```python
from build123d import *

# Parameters (mm, degrees)
EXTRUDE_1_DEPTH     = 4
SKETCH_3_R          = 5.9
EXTRUDE_2_DEPTH     = 1
SKETCH_4_R          = 2.15
CUT_EXTRUDE_1_DEPTH = 10.727281223
CHAMFER_1_SIZE      = 0.5


with BuildPart() as part:
    # Sketch 1 → Extrude 1 (new body)
    with BuildSketch(Plane.XY):
        Polygon((0, 4.618802154), (-4, 2.309401077), (-4, -2.309401077), (0, -4.618802154), (4, -2.309401077), (4, 2.309401077), align=None)
    extrude(amount=-EXTRUDE_1_DEPTH)

    # Sketch 2 → Cut-Revolve 1 (revolve, cut)
    with BuildSketch(Plane(origin=(0, 0, 0), x_dir=(0, 0, -1), z_dir=(1, 0, 0))):
        Polygon((0, 4.618802154), (0.35726559, 4.618802154), (0, 4), align=None)
        Polygon((4, 4), (3.64273441, 4.618802154), (4, 4.618802154), align=None)
    revolve(axis=Axis((0, 0, 0), (0, 0, -1)), mode=Mode.SUBTRACT)

    # Sketch 3 → Extrude 2 (add)
    with BuildSketch(Plane.XY):
        Circle(SKETCH_3_R)
    extrude(amount=EXTRUDE_2_DEPTH)

    # Sketch 4 → Cut-Extrude 1 (cut, through all)
    with BuildSketch(Plane(origin=(0, 0, -4), x_dir=(-1, 0, 0), z_dir=(0, 0, -1))):
        Circle(SKETCH_4_R)
    extrude(amount=-CUT_EXTRUDE_1_DEPTH, mode=Mode.SUBTRACT)

    # Chamfer 1
    chamfer_1_edges = [part.edges().sort_by_distance(p)[0] for p in [
        (2.15, 0, 1),
        (2.15, 0, -4),
    ]]
    chamfer(chamfer_1_edges, length=CHAMFER_1_SIZE)


solid = part.part
```
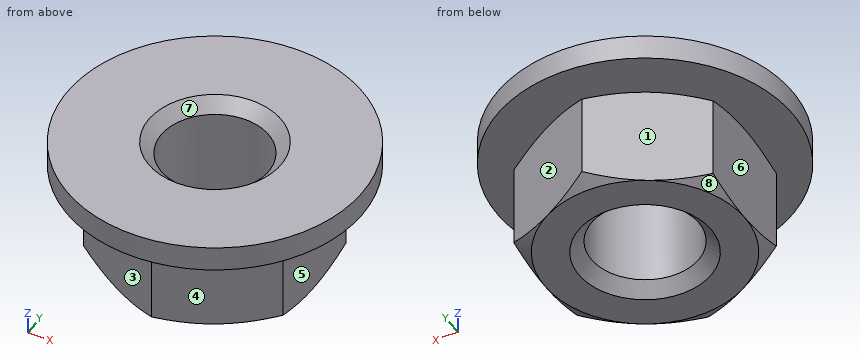
Could you check a few things on this model? Use its own coordinates, in mm. Face numbers are marked on the shaded views. A direction names the side the tool comes from. Coordinates: 2 decimals unless noted, no trailing zeros. Loops run counter-clockwise (first coordinate to the right, second up) from the corner with the lowest first, then second, coordinate; pieces in that order, holes last. Notation, with made-up numbers: M 86.25,35 L 114.25,35 A27 cw 114.25,67 Z; hole C -16.5,40 d3. An arc over 180 degrees is marked long. Put each result on its own line as item: value. Start each with the question number.
(1) I need wall thicknesses on line 1 (Z direction, x = 4.5, y = -1.25); line 2 (Y direction, x = 0.25, z = -2.05); line 3 (X direction, y = -1, z = -2.9). Which ranges of each line are inside material? Lowest first, please. Write a range as from..to.
(2) Suppose I cut it at C-C on z = 0.35. Please give me the cut outline in (x, y), then the cut area to 3 significant figures.
(3) Suppose I cut it at B-B on x = 5. Please give me the cut outline in (y, z).
(4) Will these pins go through, and if not, where does the flat tip stop? P1, Ø3, axis at y = 1, z = -3, coming from the +X side; P2, Ø1.5, axis at x = -1.5, y = -0.5, coming from the -Z side; P3, Ø1.2, axis at y = -0.5, z = -2.5, coming from the -X side.
(5) For the marked faces 1, 2, 3, 4 and 5, which set-ups out of +Z, -Z, +X, -X, +Y, -Y let a thin tool reach every point of the face, with its end or its side?
(6) Suppose I cut it at A-A on z = -1.8. Please give me the cut outline in (x, y).
(7) Thinking about a two-plate mould opening in Y: for the marked faces 6, 7 and 8, which applies, pulls with the +Y half, pulls with the -Y half, needs draft (parallel to the pull), parting line crosses it, or undercut?
Solutions:
1. line 1: z = 0..1
1. line 2: y = -4.47..-2.14, 2.14..4.47
1. line 3: x = -4..-1.9, 1.9..4
2. outline: C 0,0 d11.8; hole C 0,0 d4.3
2. area: 94.8 mm2
3. outline: M -3.13,0 L 3.13,0 L 3.13,1 L -3.13,1 Z
4. P1: stops at x = 4
4. P2: stops at z = -3.68
4. P3: stops at x = -4
5. face 1: -Z, -X, +Y
5. face 2: -Z, +X, +Y
5. face 3: -Z, -X, -Y
5. face 4: -Z, +X, -Y
5. face 5: -Z, +X, +Y, -Y
6. outline: M -4,-2.31 L 0,-4.62 L 4,-2.31 L 4,2.31 L 0,4.62 L -4,2.31 Z; hole C 0,0 d4.3
7. face 6: needs draft
7. face 7: undercut
7. face 8: pulls with the +Y half
